Autodesk Inventor part; units mm, degrees
ref_plane "YZ Plane" through (0, 0, 0) normal (1, 0, 0) x (0, 1, 0)
ref_plane "XZ Plane" through (0, 0, 0) normal (0, 1, 0) x (-1, 0, 0)
ref_plane "XY Plane" through (0, 0, 0) normal (0, 0, 1) x (1, 0, 0)
sketch "スケッチ1" plane through (0, 0, 0) normal (0, 0, 1) x (1, 0, 0)
  circle A0 centre (0, 0) radius 3
  dimension "d0" = 6
extrude "押し出し1" add sketch "スケッチ1" along normal blind 55
sketch "スケッチ2" plane through (0, 0, 55) normal (0, 0, 1) x (1, 0, 0)
  circle A0 centre (0, 0) radius 1.5
  dimension "d3" = 3
extrude "押し出し2" cut sketch "スケッチ2" against normal blind 6
sketch "スケッチ3" plane through (0, 0, 0) normal (0, 0, -1) x (-1, 0, 0)
  circle A0 centre (0, 0) radius 1.5
  circle A1 centre (0, 0) radius 1.5
  dimension "d6" = 3
extrude "押し出し3" cut sketch "スケッチ3" against normal blind 6
properties part number "スペーサーm3-55" material "アルミニウム 2014-T4"
Here's how the part is built. I have some questions about the finished solid (model axes, mm). A direction names the side the tool comes from. Coordinates: 2 decimals unless noted, no trailing zeros. Write each loop counter-clockwise with the first axis right and the second up, starting at its lowest first coordinate (ties: lowest second). Pieces come first, ordered by that corner, then holes.
1) Thinking about a two-plate mould opening in Y: for faces 4 (the face through (-1.5, 0.07, 52.04)), 5 (the face through (1.3, -1.3, 0)), 6 (the face through (-3, 0, 27)), which applies, +Y half, -Y half, draft (parallel to the pull), parting line (faces both ways), or undercut?
Filled in:
face 4: undercut
face 5: draft
face 6: parting line
2) If we section it at C-C (z = 28): List the corners of the cut face in (x, y) for me, plus the area to 3 significant figures.
Filled in:
outline: circle Ø6 at (0, 0)
area: 28.3 mm2
3) Which directions (+Z, -Z, +X, -X, +Y, -Y) give clear straight access to the entire face, cutting with the end or side of a thin tool? Please do faces 1 (the face through (1.5, 0.07, 2.96)), 2 (the face through (0, 0, 49)), 3 (the face through (1.3, -1.3, 55)).
Filled in:
face 1: -Z
face 2: +Z
face 3: +Z, +X, -X, +Y, -Y
4) If I drill on line 1 (Y direction, x = 0, z = 52.1); line 2 (Z direction, x = -0.15, y = -0.95); line 3 (Y direction, x = -1.25, z = 4.5), over which ranges is the centre line in solid material (lowest first)?
Filled in:
line 1: y = -3 to -1.5, 1.5 to 3
line 2: z = 6 to 49
line 3: y = -2.73 to -0.83, 0.83 to 2.73
5) I'm going to push flat-ended pins straight in: pin 1 (3 mm diameter, centred on y = -2, z = 19, fed in from -X); pin 2 (2.5 mm diameter, centred on x = 0, y = 0, fed in from +Z); pin 3 (2 mm diameter, centred on x = -1.5, z = 32, fed in from -Y). Where does each tip first touch, or does it pass through?
Filled in:
pin 1: stops at x = -2.96
pin 2: stops at z = 49
pin 3: stops at y = -2.96
6) If we section it at D-D (y = -2.2): List the corners of the cut face in (x, z) for me, plus the area to 3 significant figures.
Filled in:
outline: (-2.04, 0) - (2.04, 0) - (2.04, 55) - (-2.04, 55) - close
area: 224 mm2
7) If we section it at A-A (x = 0): List the corners of the cut face in (y, z) for me, plus the area to 3 significant figures.
Filled in:
outline: (-3, 0) - (-1.5, 0) - (-1.5, 6) - (1.5, 6) - (1.5, 0) - (3, 0) - (3, 55) - (1.5, 55) - (1.5, 49) - (-1.5, 49) - (-1.5, 55) - (-3, 55) - close
area: 294 mm2
